Drawing for the job (mm, zero at the part's lowest x, y, z). A direction names the side the tool comes from. Round coordinates to 2 decimals unless told otherwise and drop trailing zeros. Write each loop counter-clockwise with the first axis right and the second up, starting at its lowest first coordinate (ties: lowest second). Pieces come first, ordered by that corner, then holes. Notation, with made-up numbers: (-32, 40.5) - (-25, 40.5) arc R27 cw to (-25, 68.5) - close; hole circle Ø5 at (44, 1.5). An arc over 180 degrees is marked (long way). One line per question, with ' | ' between items.
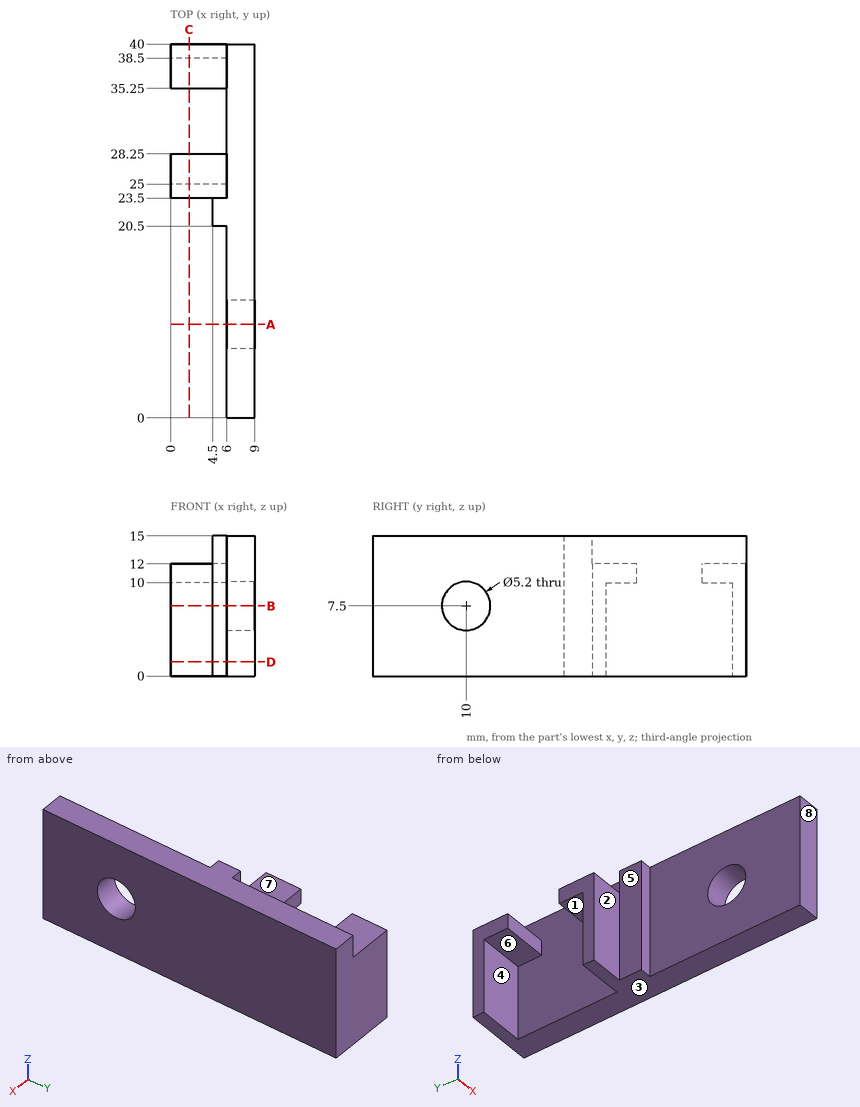
Q1. Pull direction Y, two halves, no side cores. Call the marked faces 1, 2, 3 and 4: +Y half, -Y half, draft (parallel to the pull), parting line (faces both ways), or undercut.
Found:
face 1: undercut | face 2: -Y half | face 3: draft | face 4: undercut
Q2. Drill centre lines: L1, parallel to Y at x = 8.15, z = 7.5; L2, parallel to Y at x = 1.5, z = 5.25; L3, parallel to X at y = 20, z = 10. Where is each one in solid material? Low to high. Write a range as from..to.
Found:
L1: 0..7.4, 12.6..40 | L2: 23.5..25, 38.5..40 | L3: 6..9
Q3. Which spindle directions (+Z, -Z, +X, -X, +Y, -Y) get a long thin tool onto all of the face, cutting with end or side? Do the marked faces 5, 6, 7 and 8. Say none if no direction does.
Found:
face 5: +Z, -Z, -X, -Y | face 6: -Z, -X | face 7: +Z, -X, +Y | face 8: +Z, -Z, +X, -X, -Y
Q4. Drop flat-ended pins along their axis: pin 1 (1 mm diameter, centred on x = 4, y = 36, fed in from -Z); pin 2 (1.4 mm diameter, centred on x = 3.5, y = 38.5, fed in from +Z); pin 3 (2.5 mm diameter, centred on y = 22, z = 4.5, fed in from -X); pin 4 (4 mm diameter, centred on y = 10, z = 7.5, fed in from +X). Give the stop position or say it passes through.
Found:
pin 1: z = 10 | pin 2: z = 12 | pin 3: x = 4.5 | pin 4: through
Q5. Saw through at B-B, the plane z = 7.5. List the corners of the cut face in (x, y).
Found:
outline: (0, 23.5) - (4.5, 23.5) - (4.5, 20.5) - (6, 20.5) - (6, 12.6) - (9, 12.6) - (9, 40) - (0, 40) - (0, 38.5) - (6, 38.5) - (6, 25) - (0, 25) - close; (6, 0) - (9, 0) - (9, 7.4) - (6, 7.4) - close
Q6. Saw through at C-C, the plane x = 2. List the corners of the cut face in (y, z).
Found:
outline: (23.5, 0) - (25, 0) - (25, 10) - (28.25, 10) - (28.25, 12) - (23.5, 12) - close; (35.25, 10) - (38.5, 10) - (38.5, 0) - (40, 0) - (40, 12) - (35.25, 12) - close
Q7. Saw through at A-A, the plane y = 10. List the corners of the cut face in (x, z).
Found:
outline: (6, 0) - (9, 0) - (9, 4.9) - (6, 4.9) - close; (6, 10.1) - (9, 10.1) - (9, 15) - (6, 15) - close
Q8. Saw through at D-D, the plane z = 1.5. List the corners of the cut face in (x, y).
Found:
outline: (0, 23.5) - (4.5, 23.5) - (4.5, 20.5) - (6, 20.5) - (6, 0) - (9, 0) - (9, 40) - (0, 40) - (0, 38.5) - (6, 38.5) - (6, 25) - (0, 25) - close
